```python
from build123d import *

# Parameters (mm, degrees)
F1_DEPTH = 152.4
F3_R     = 165.1
F4_DEPTH = 152.4
F6_R     = 165.1
F7_DEPTH = 152.4


with BuildPart() as f1:
    # F0 (on Top) → F1 (new body)
    with BuildSketch(Plane.XY):
        with BuildLine():
            Line((0, 635), (0, 0))
            Line((0, 0), (1752.6, 0))
            Line((1752.6, 0), (1752.6, 152.4))
            Line((1752.6, 152.4), (1040.841937, 152.4))
            ThreePointArc((1040.841937, 152.4), (875.741937, 317.5), (1040.841937, 482.6))
            Line((1040.841937, 482.6), (1752.6, 482.6))
            Line((1752.6, 482.6), (1752.6, 635))
            Line((1752.6, 635), (0, 635))
        make_face()
    extrude(amount=F1_DEPTH)

    # F3 (on offset) → F4 (join)
    with BuildSketch(Plane.YZ.offset(152.4)):
        with BuildLine():
            Line((0, 609.6), (0, 152.4))
            Line((0, 152.4), (635, 152.4))
            Line((635, 152.4), (635, 609.6))
            ThreePointArc((635, 609.6), (317.5, 927.1), (0, 609.6))
        make_face()
        with Locations((317.5, 609.6)):
            Circle(F3_R, mode=Mode.SUBTRACT)
    extrude(amount=-F4_DEPTH)

    # F6 (on offset) → F7 (join)
    with BuildSketch(Plane.XZ.offset(-635)):
        with BuildLine():
            Line((635, 0), (0, 0))
            Line((0, 0), (0, -304.8))
            ThreePointArc((0, -304.8), (317.5, -622.3), (635, -304.8))
            Line((635, -304.8), (635, 0))
        make_face()
        with Locations((317.5, -304.8)):
            Circle(F6_R, mode=Mode.SUBTRACT)
    extrude(amount=F7_DEPTH)


solid = f1.part
```
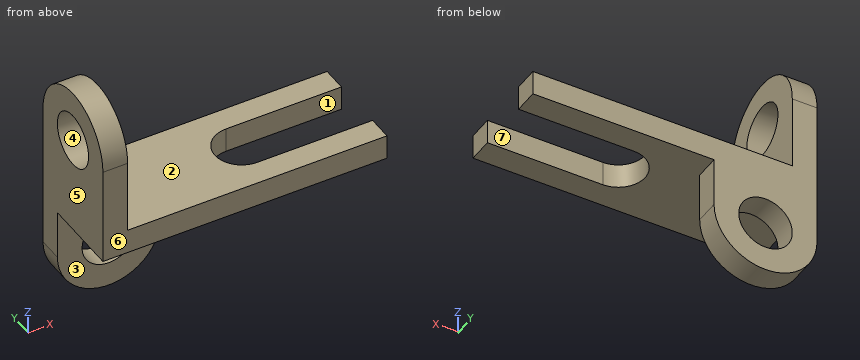
Build history of the part. All positions in model axes, mm. Face numbers are marked on the shaded views. A direction names the side the tool comes from. Give positions to 0.01 mm unless a question says otherwise; leave off trailing zeros. Order: outer loops, then holes, each group sorted by start corner. A loop starts at its lowest first (then second) coordinate and runs counter-clockwise, first axis right, second up. Notation, with made-up numbers: M 44,61 L 98,61 A6 ccw 98,70 Z; hole C 57.5,31.5 d6. An arc over 180 degrees is marked long. Return JSON: item names as keys, results as strings.
Q1. Band-saw the part on A-A (x = 1625.5). Give the cut face in (y, z).
Answer list:
{"outline": "M 0,0 L 152.4,0 L 152.4,152.4 L 0,152.4 Z; M 482.6,0 L 635,0 L 635,152.4 L 482.6,152.4 Z"}
Q2. Wall check: probe 1 along Y at (x, z) = (1557.5, 95.5); probe 2 along Z at (x, y) = (107, 317.5). Give the ranges that are in metal, low to high. Write a range as from..to.
Answer list:
{"probe 1": "y = 0..152.4, 482.6..635", "probe 2": "z = 0..444.5, 774.7..927.1"}
Q3. Flat gauge pins, fed straight in: pin 1 (3 mm diameter, centred on y = 400, z = 109.5, fed in from +X); pin 2 (12 mm diameter, centred on y = 157.5, z = 229.5, fed in from -X); pin 3 (5 mm diameter, centred on x = 822, y = 253, fed in from +Z); pin 4 (8 mm diameter, centred on x = 821, y = 331.5, fed in from -Z). Where does each tip first touch, or does it go through?
Answer list:
{"pin 1": "stops at x = 898.71", "pin 2": "stops at x = 0", "pin 3": "stops at z = 152.4", "pin 4": "stops at z = 0"}
Q4. Band-saw the part on D-D (x = 317.5). Give the cut face in (y, z).
Answer list:
{"outline": "M 0,0 L 482.6,0 L 482.6,-139.7 L 635,-139.7 L 635,152.4 L 0,152.4 Z; M 482.6,-622.3 L 635,-622.3 L 635,-469.9 L 482.6,-469.9 Z"}
Q5. 3-axis set-ups, long thin cutter, end or side, ignore diameter. For the marked faces 1, 2 and 3: which of +Z, -Z, +X, -X, +Y, -Y reach the whole face in a straight line?
Answer list:
{"face 1": "+Z, -Z, +X", "face 2": "+Z, +X, +Y, -Y", "face 3": "-Z, +X, -X, -Y"}
Q6. Band-saw the part on B-B (y = 373). Give the cut face in (x, z), then the cut area to 3 significant figures.
Answer list:
{"outline": "M 0,0 L 885.35,0 L 885.35,152.4 L 152.4,152.4 L 152.4,454.11 L 0,454.11 Z; M 0,765.09 L 152.4,765.09 L 152.4,922.21 L 0,922.21 Z", "area": "205,000 mm^2"}
Q7. Two-plate mould, pull along Y, no slides. Class the marked faces 4, 5, 6 and 7: pulls with the +Y half, pulls with the -Y half, needs draft (parallel to the pull), parting line crosses it, or undercut.
Answer list:
{"face 4": "undercut", "face 5": "needs draft", "face 6": "pulls with the -Y half", "face 7": "undercut"}
Q8. Band-saw the part on C-C (z = -190.5). Give the cut face in (x, y), then the cut area to 3 significant figures.
Answer list:
{"outline": "M 0,482.6 L 198.36,482.6 L 198.36,635 L 0,635 Z; M 436.64,482.6 L 635,482.6 L 635,635 L 436.64,635 Z", "area": "60,500 mm^2"}
